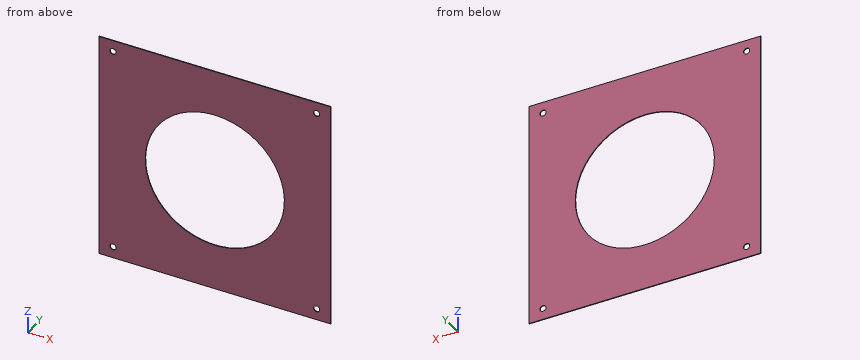
from build123d import *

# Parameters (mm, degrees)
SKETCH1_W           = 254
SKETCH1_H           = 254
SKETCH1_R           = 3.3782
BOSS_EXTRUDE1_DEPTH = 0.79375
SKETCH2_R           = 76.2
CUT_EXTRUDE1_DEPTH  = 0.79375


with BuildPart() as part:
    # Sketch1 → Boss-Extrude1 (new body)
    with BuildSketch(Plane(origin=(0, 0, 0), x_dir=(1, 0, 0), z_dir=(0, 1, 0))):
        Rectangle(SKETCH1_W, SKETCH1_H)
        with Locations(Location((-111.506, 114.3, 0), (0, 0, 270))):
            Circle(SKETCH1_R, mode=Mode.SUBTRACT)
        with Locations(Location((111.506, 114.3, 0), (0, 0, 270))):
            Circle(SKETCH1_R, mode=Mode.SUBTRACT)
        with Locations(Location((111.506, -114.3, 0), (0, 0, 270))):
            Circle(SKETCH1_R, mode=Mode.SUBTRACT)
        with Locations(Location((-111.506, -114.3, 0), (0, 0, 270))):
            Circle(SKETCH1_R, mode=Mode.SUBTRACT)
    extrude(amount=BOSS_EXTRUDE1_DEPTH)

    # Sketch2 → Cut-Extrude1 (cut)
    with BuildSketch(Plane(origin=(0, 0.79375, 0), x_dir=(1, 0, 0), z_dir=(0, 1, 0))):
        with Locations(Location((0, 0, 0), (0, 0, 270))):
            Circle(SKETCH2_R)
    extrude(amount=-CUT_EXTRUDE1_DEPTH, mode=Mode.SUBTRACT)


solid = part.part
Input: part model. Units: mm. Frame: model coordinates. Round coordinates to 2 decimals unless told otherwise and drop trailing zeros. Order: outer loops, then holes, each group sorted by start corner. A loop starts at its lowest first (then second) coordinate and runs counter-clockwise, first axis right, second up. Notation, with made-up numbers: (25.5, 39) - (73.5, 39) arc R28 ccw to (73.5, 66) - close; hole circle Ø8 at (28, 31.25). An arc over 180 degrees is marked (long way). Use a Markdown table: item, result.
1. Material intervals for probe 1 along X at (y, z) = (0.55, 114.3); probe 2 along X at (y, z) = (0.4, 1.5); probe 3 along Z at (x, y) = (0.5, 0.55), sorted ascending.
Evaluation:
| item | result |
|---|---|
| probe 1 | -127 to -114.88, -108.13 to 108.13, 114.88 to 127 |
| probe 2 | -127 to -76.19, 76.19 to 127 |
| probe 3 | -127 to -76.2, 76.2 to 127 |
2. Section C-C on z = -114.3. Return the cut outline in (x, y), then the cut area to 3 significant figures.
Evaluation:
| item | result |
|---|---|
| outline | (-127, 0) - (-114.88, 0) - (-114.88, 0.79) - (-127, 0.79) - close; (-108.13, 0) - (108.13, 0) - (108.13, 0.79) - (-108.13, 0.79) - close; (114.88, 0) - (127, 0) - (127, 0.79) - (114.88, 0.79) - close |
| area | 191 mm^2 |
3. Section B-B on x = 0. Return the cut outline in (y, z), then the cut area to 3 significant figures.
Evaluation:
| item | result |
|---|---|
| outline | (0, -127) - (0.79, -127) - (0.79, -76.2) - (0, -76.2) - close; (0, 76.2) - (0.79, 76.2) - (0.79, 127) - (0, 127) - close |
| area | 80.6 mm^2 |
4. Section A-A on z = 15. Return the cut outline in (x, y), then the cut area to 3 significant figures.
Evaluation:
| item | result |
|---|---|
| outline | (-127, 0) - (-74.71, 0) - (-74.71, 0.79) - (-127, 0.79) - close; (74.71, 0) - (127, 0) - (127, 0.79) - (74.71, 0.79) - close |
| area | 83.0 mm^2 |
5. First-contact query: pin 1 (4 mm diameter, centred on x = -111.506, z = 114.3, fed in from -Y). Flat tip, straight axial feed; report the tip coordinate or a pass-through.
Evaluation:
| item | result |
|---|---|
| pin 1 | through |
6. Section D-D on y = 0.45. Return the cut outline in (x, z).
Evaluation:
| item | result |
|---|---|
| outline | (-127, -127) - (127, -127) - (127, 127) - (-127, 127) - close; hole circle Ø6.76 at (-111.51, -114.3); hole circle Ø6.76 at (-111.51, 114.3); hole circle Ø152.4 at (0, 0); hole circle Ø6.76 at (111.51, -114.3); hole circle Ø6.76 at (111.51, 114.3) |
